Verification items for the finished model (mm, model axes). A direction names the side the tool comes from. Give positions to 0.01 mm unless a question says otherwise; leave off trailing zeros. Order: outer loops, then holes, each group sorted by start corner. A loop starts at its lowest first (then second) coordinate and runs counter-clockwise, first axis right, second up. Notation, with made-up numbers: (10.5, 54) - (14.5, 54) arc R12 ccw to (14.5, 67) - close; hole circle Ø5 at (58.5, -10.75). An arc over 180 degrees is marked (long way). Answer as a JSON object with one key per item and string values. Group by question number.
(1) Access from +Z, -Z, +X, -X, +Y, -Y to the whole of each face (thin tool, end or side, straight path). Record for faces 4 (the face through (-106.93, -0.63, 40.34)), 5 (the face through (-102.926, -3.399, 38.949)).
(2) Depth check by flat-ended pin: pin 1 Ø1.7 at (x, z) = (-105, 41) entering from +Y; pin 2 Ø1 at (x, z) = (-103, 29.5) entering from +Y; pin 3 Ø2.5 at (x, z) = (-104.26, 39.5) entering from +Y. Enter the tip coordinate at first touch or a pass-through.
(3) Mould release check, pull along Z, two halves, no side actions. Record for faces 1 (the face through (-105, -1.27, 38)), 2 (the face through (-104, -3, 42.399)), 3 (the face through (-104.4, 0, 36.5)): +Z half, -Z half, draft (parallel to the pull), parting line (faces both ways), or undercut.
(4) Section check D-D (y = -1.9). Record the boundary of the cut face in (x, z), then the cut area to 3 significant figures.
(5) Section check C-C (x = -107.5). Record the boundary of the cut face in (y, z).
(6) Section check A-A (x = -105). Record the boundary of the cut face in (y, z).
(7) Thickness scan on line 1 (Y direction, x = -104.25, z = 37.75); line 2 (Z direction, x = -105.25, y = -2); line 3 (Z direction, x = -105.5, y = -5.1). Record the ranges inside material, lowest first.
(8) Section check B-B (z = 41.25). Record the boundary of the cut face in (x, y).
```python
from build123d import *

# Parameters (mm, degrees)
F0_W     = 7.874
F0_H     = 15.24
F0_R     = 1.4478
F1_DEPTH = 5.588
F2_R     = 2.794
F3_DEPTH = 1.27
F5_DEPTH = 25.4


# Not quite as in the source:
# - a feature names something its author has since deleted; it is built from what else it names


with BuildPart() as f1:
    # F0 (on Front) → F1 (new body)
    with BuildSketch(Plane.XZ):
        with Locations((-104.3903227065, 34.7791743618)):
            Rectangle(F0_W, F0_H)
        with Locations((-104.2633227065, 39.5035743618)):
            Circle(F0_R, mode=Mode.SUBTRACT)
    extrude(amount=F1_DEPTH)

    # F2 (on face) → F3 (cut)
    with BuildSketch(Plane(origin=(0, 0, 0), x_dir=(-1, 0, 0), z_dir=(0, 1, 0))):
        with Locations((104.2633227065, 39.5035743618)):
            Circle(F2_R)
    extrude(amount=-F3_DEPTH, mode=Mode.SUBTRACT)

    # F4 (on face) → F5 (cut)
    with BuildSketch(Plane.YZ.offset(-100.4533227065)):
        Polygon((0, 34.1825485229), (-0.8814302273, 27.1591743618), (0, 27.1591743618), align=None)
    extrude(amount=-F5_DEPTH, mode=Mode.SUBTRACT)


solid = f1.part
```
Solutions:
{
 "1": {"face 4": "+Y", "face 5": "+Y, -Y"},
 "2": {"pin 1": "stops at y = -1.27", "pin 2": "stops at y = -0.52", "pin 3": "passes through"},
 "3": {"face 1": "undercut", "face 2": "+Z half", "face 3": "draft"},
 "4": {"outline": "(-108.33, 27.16) - (-100.45, 27.16) - (-100.45, 42.4) - (-108.33, 42.4) - close; hole circle Ø2.9 at (-104.26, 39.5)", "area": "113 mm2"},
 "5": {"outline": "(-5.59, 27.16) - (-0.88, 27.16) - (0, 34.18) - (0, 42.4) - (-5.59, 42.4) - close"},
 "6": {"outline": "(-5.59, 27.16) - (-0.88, 27.16) - (0, 34.18) - (0, 36.81) - (-1.27, 36.81) - (-1.27, 38.26) - (-5.59, 38.26) - close; (-5.59, 40.75) - (-1.27, 40.75) - (-1.27, 42.2) - (0, 42.2) - (0, 42.4) - (-5.59, 42.4) - close"},
 "7": {"line 1": "y = -5.59 to -1.27", "line 2": "z = 27.16 to 38.44, 40.56 to 42.4", "line 3": "z = 27.16 to 38.75, 40.26 to 42.4"},
 "8": {"outline": "(-108.33, -5.59) - (-100.45, -5.59) - (-100.45, 0) - (-102.08, 0) - (-102.08, -1.27) - (-106.44, -1.27) - (-106.44, 0) - (-108.33, 0) - close"}
}
